Model file for the job. Use its own axes, mm. Round coordinates to 2 decimals unless told otherwise and drop trailing zeros. Write each loop counter-clockwise with the first axis right and the second up, starting at its lowest first coordinate (ties: lowest second). Pieces come first, ordered by that corner, then holes. Notation, with made-up numbers: (39.25, 84) - (91.25, 84) arc R13 ccw to (91.25, 89) - close; hole circle Ø9 at (-2.75, 28.25). An arc over 180 degrees is marked (long way). Answer as a JSON object with one key per item and string values. Group by question number.
from build123d import *

# Parameters (mm, degrees)
BOSS_EXTRUDE1_DEPTH     = 3
SKETCH2_W               = 27.727272727
SKETCH2_H               = 3
SKETCH2_W_2             = 3
SKETCH2_H_2             = 18
SKETCH2_H_3             = 9
SKETCH2_W_3             = 23.343342349
SKETCH2_W_4             = 23.34334235
SKETCH2_W_5             = 6
CUT_EXTRUDE1_DEPTH      = 1
CUT_EXTRUDE1_DEPTH_BACK = 4
SKETCH3_W               = 3.2
SKETCH3_H               = 10.5
SKETCH3_W_2             = 5.2
SKETCH3_H_2             = 2.5
CUT_EXTRUDE2_DEPTH      = 1
CUT_EXTRUDE2_DEPTH_BACK = 4
FILLET1_R               = 2.5
SKETCH4_R               = 5
BOSS_EXTRUDE2_DEPTH     = 3
FILLET2_R               = 2.5
SKETCH5_R               = 2.5
SKETCH5_R_2             = 2
SKETCH5_R_3             = 10
SKETCH5_W               = 3.05
SKETCH5_H               = 15
CUT_EXTRUDE3_DEPTH      = 1
CUT_EXTRUDE3_DEPTH_BACK = 4


with BuildPart() as part:
    # Sketch1 → Boss-Extrude1 (new body)
    with BuildSketch(Plane(origin=(0, 0, 0), x_dir=(0, 0, -1), z_dir=(1, 0, 0))):
        with BuildLine():
            Line((-152.5, 33), (152.5, 33))
            Line((152.5, 33), (152.5, 23))
            Line((152.5, 23), (107.5, 23))
            ThreePointArc((107.5, 23), (72.144660941, 8.355339059), (57.5, -27))
            Line((57.5, -27), (57.5, -33))
            Line((57.5, -33), (-152.5, -33))
            Line((-152.5, -33), (-152.5, 33))
        make_face()
    extrude(amount=BOSS_EXTRUDE1_DEPTH)

    # Sketch2 → Cut-Extrude1 (cut, two sides)
    with BuildSketch(Plane(origin=(3, 0, 0), x_dir=(0, 0, -1), z_dir=(1, 0, 0))) as cut_extrude1_sk:
        with Locations((27.727272728, 31.5)):
            Rectangle(SKETCH2_W, SKETCH2_H)
        with Locations((83.181818182, 31.5)):
            Rectangle(SKETCH2_W, SKETCH2_H)
        with Locations((-138.636363636, 31.5)):
            Rectangle(SKETCH2_W, SKETCH2_H)
        with Locations((-83.181818182, 31.5)):
            Rectangle(SKETCH2_W, SKETCH2_H)
        with Locations((-27.727272728, 31.5)):
            Rectangle(SKETCH2_W, SKETCH2_H)
        with Locations((-151, 3)):
            Rectangle(SKETCH2_W_2, SKETCH2_H_2)
        with Locations((-151, -28.5)):
            Rectangle(SKETCH2_W_2, SKETCH2_H_3)
        with Locations((-117.484986475, -28.5)):
            Rectangle(SKETCH2_W_3, SKETCH2_H)
        with Locations((-70.798301777, -28.5)):
            Rectangle(SKETCH2_W_3, SKETCH2_H)
        with Locations((22.575067622, -28.5)):
            Rectangle(SKETCH2_W_4, SKETCH2_H)
        with Locations((149.5, 31.5)):
            Rectangle(SKETCH2_W_5, SKETCH2_H)
        with Locations((-24.111617078, -28.5)):
            Rectangle(SKETCH2_W_3, SKETCH2_H)
    extrude(amount=CUT_EXTRUDE1_DEPTH, mode=Mode.SUBTRACT)
    extrude(cut_extrude1_sk.sketch, amount=-CUT_EXTRUDE1_DEPTH_BACK, mode=Mode.SUBTRACT)

    # Sketch3 → Cut-Extrude2 (cut, two sides)
    with BuildSketch(Plane(origin=(3, 0, 0), x_dir=(0, 0, -1), z_dir=(1, 0, 0))) as cut_extrude2_sk:
        with Locations((-110.909090909, 27.75)):
            Rectangle(SKETCH3_W, SKETCH3_H)
        with Locations((55.454545455, 27.75)):
            Rectangle(SKETCH3_W, SKETCH3_H)
        with Locations((55.454545455, 28.575)):
            Rectangle(SKETCH3_W_2, SKETCH3_H_2)
        with Locations((-110.909090909, 28.575)):
            Rectangle(SKETCH3_W_2, SKETCH3_H_2)
    extrude(amount=CUT_EXTRUDE2_DEPTH, mode=Mode.SUBTRACT)
    extrude(cut_extrude2_sk.sketch, amount=-CUT_EXTRUDE2_DEPTH_BACK, mode=Mode.SUBTRACT)

    # Fillet1
    fillet1_edges = [part.edges().sort_by_distance(p)[0] for p in [
        (1.5, -33, -57.5),
    ]]
    fillet(fillet1_edges, radius=FILLET1_R)

    # Sketch4 → Boss-Extrude2 (add)
    with BuildSketch(Plane(origin=(0, 0, 0), x_dir=(0, 0, -1), z_dir=(1, 0, 0))):
        with BuildLine():
            Line((-55.454545455, 30), (-55.454545455, 177))
            ThreePointArc((-55.454545455, 177), (-38.304207087, 196.795944751), (-16.266602596, 182.641174423))
            Line((-16.266602596, 182.641174423), (27.727272727, 33))
            Line((27.727272727, 33), (27.727272727, 30))
            Line((27.727272727, 30), (-55.454545455, 30))
        make_face()
        with Locations((-35.454545455, 177)):
            Circle(SKETCH4_R, mode=Mode.SUBTRACT)
        Polygon((-30.454545455, 55), (-4.798665146, 55), (-30.454545455, 142.266148573), align=None, mode=Mode.SUBTRACT)
    extrude(amount=BOSS_EXTRUDE2_DEPTH)

    # Fillet2
    fillet2_edges = [part.edges().sort_by_distance(p)[0] for p in [
        (1.5, 55, 30.454545455),
        (1.5, 55, 4.798665146),
        (1.5, 142.266148573, 30.454545455),
    ]]
    fillet(fillet2_edges, radius=FILLET2_R)

    # Sketch5 → Cut-Extrude3 (cut, two sides)
    with BuildSketch(Plane(origin=(3, 0, 0), x_dir=(0, 0, -1), z_dir=(1, 0, 0))) as cut_extrude3_sk:
        with Locations((10.227172727, 31.5)):
            Circle(SKETCH5_R)
        with Locations((-35.454545455, 152)):
            Circle(SKETCH5_R)
        with Locations((-8.454545455, 46)):
            Circle(SKETCH5_R_2)
        with Locations((10, 0)):
            Circle(SKETCH5_R_3)
        Polygon((-3.003684653, 87.804874126), (-7.23456547, 102.195831269), (-4.308404184, 103.056110369), (-0.077523367, 88.665153225), align=None)
        with Locations((-42.954545455, 91.19961143)):
            Rectangle(SKETCH5_W, SKETCH5_H)
    extrude(amount=CUT_EXTRUDE3_DEPTH, mode=Mode.SUBTRACT)
    extrude(cut_extrude3_sk.sketch, amount=-CUT_EXTRUDE3_DEPTH_BACK, mode=Mode.SUBTRACT)


solid = part.part
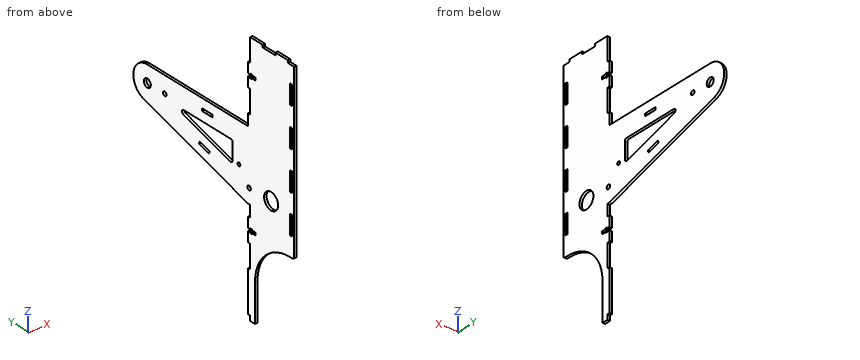
(1) Slice it at C-C (x = 2.5). Count the separate pieces of the cut face and the enclosed holes in it, then the cut area to 3 significant figures.
(2) Slice it at A-A (z = -31). Write the cut outline in (x, y), then the cut area to 3 significant figures.
(3) Drill centre lines: line 1 (Y direction, x = 0.9, z = 119); line 2 (Y direction, x = 1.55, z = -32.5); line 3 (Y direction, x = 1.55, z = -107). Where is each one in solid material? Low to high. Write a range as from..to.
(4) Slice it at B-B (y = 0). Write the cut outline in (x, z).
(5) Flat gauge pins, fed straight in: pin 1 (1.5 mm diameter, centred on x = 1, z = 102, fed in from +Y); pin 2 (0.9 mm diameter, centred on x = 2, y = 96.5, fed in from -Z); pin 3 (1.5 mm diameter, centred on x = 1.5, y = 41, fed in from +Z). Where does each tip first touch, or does it go through?
(6) Slice it at D-D (z = -124). Write the cut outline in (x, y), then the cut area to 3 significant figures.
Answer:
{
 "1": {"separate pieces": "1", "enclosed holes": "12", "area": "22,500 mm²"},
 "2": {"outline": "(0, -33) - (3, -33) - (3, -30) - (0, -30) - close; (0, -27) - (3, -27) - (3, 30) - (0, 30) - close", "area": "180 mm²"},
 "3": {"line 1": "-33..-30, -27..33", "line 2": "-33..-30, -27..30", "line 3": "23..33"},
 "4": {"outline": "(0, -65.42) - (3, -65.42) - (3, -20) - (0, -20) - close; (0, 0) - (3, 0) - (3, 149.5) - (0, 149.5) - close"},
 "5": {"pin 1": "y = 33", "pin 2": "z = -9.19", "pin 3": "z = 55.45"},
 "6": {"outline": "(0, 23) - (3, 23) - (3, 33) - (0, 33) - close", "area": "30.0 mm²"}
}
